Source: CAD feature listing. Evaluate the final solid. Frame: model axes, mm. A direction names the side the tool comes from. Coordinates: 2 decimals unless noted, no trailing zeros. Write each loop counter-clockwise with the first axis right and the second up, starting at its lowest first coordinate (ties: lowest second). Pieces come first, ordered by that corner, then holes. Notation, with made-up numbers: (79, 49) - (131, 49) arc R25 cw to (131, 85) - close; hole circle Ø5 at (-31.5, 29). An arc over 180 degrees is marked (long way). One line per item, written item: value.
from build123d import *

# Parameters (mm, degrees)
SKETCH1_W           = 40
SKETCH1_H           = 10
BOSS_EXTRUDE1_DEPTH = 10
SKETCH2_R           = 2
CUT_EXTRUDE1_DEPTH  = 41
CUT_EXTRUDE2_REACH  = 12
SKETCH3_R           = 0.75


with BuildPart() as part:
    # Sketch1 → Boss-Extrude1 (new body)
    with BuildSketch(Plane(origin=(0, 0, 0), x_dir=(1, 0, 0), z_dir=(0, 1, 0))):
        Rectangle(SKETCH1_W, SKETCH1_H)
    extrude(amount=BOSS_EXTRUDE1_DEPTH)

    # Sketch2 → Cut-Extrude1 (cut, through all)
    with BuildSketch(Plane(origin=(20, 0, 0), x_dir=(0, 0, -1), z_dir=(1, 0, 0))):
        with Locations((0, 4)):
            Circle(SKETCH2_R)
    extrude(amount=-CUT_EXTRUDE1_DEPTH, mode=Mode.SUBTRACT)

    # Sketch3 → Cut-Extrude2 (cut, up to next)
    with BuildSketch(Plane(origin=(0, 10, 0), x_dir=(1, 0, 0), z_dir=(0, 1, 0)), mode=Mode.PRIVATE) as cut_extrude2_sk1:
        with Locations((11, 0)):
            Circle(SKETCH3_R)
    cut_extrude2_tool1 = extrude(cut_extrude2_sk1.sketch, amount=-CUT_EXTRUDE2_REACH, mode=Mode.PRIVATE) & part.part
    add(cut_extrude2_tool1.solids().sort_by_distance((11, 10, 0))[0], mode=Mode.SUBTRACT)
    # Sketch3 → Cut-Extrude2 (cut, up to next)
    with BuildSketch(Plane(origin=(0, 10, 0), x_dir=(1, 0, 0), z_dir=(0, 1, 0)), mode=Mode.PRIVATE) as cut_extrude2_sk2:
        with Locations((6, 0)):
            Circle(SKETCH3_R)
    cut_extrude2_tool2 = extrude(cut_extrude2_sk2.sketch, amount=-CUT_EXTRUDE2_REACH, mode=Mode.PRIVATE) & part.part
    add(cut_extrude2_tool2.solids().sort_by_distance((6, 10, 0))[0], mode=Mode.SUBTRACT)
    # Sketch3 → Cut-Extrude2 (cut, up to next)
    with BuildSketch(Plane(origin=(0, 10, 0), x_dir=(1, 0, 0), z_dir=(0, 1, 0)), mode=Mode.PRIVATE) as cut_extrude2_sk3:
        with Locations((1, 0)):
            Circle(SKETCH3_R)
    cut_extrude2_tool3 = extrude(cut_extrude2_sk3.sketch, amount=-CUT_EXTRUDE2_REACH, mode=Mode.PRIVATE) & part.part
    add(cut_extrude2_tool3.solids().sort_by_distance((1, 10, 0))[0], mode=Mode.SUBTRACT)


solid = part.part
1) Reachability of faces 1 (the flat face through (-20, 6, -1)), 2 (the cylindrical face through (10.25, 7.96, -0.03)) from +Z, -Z, +X, -X, +Y, -Y: full face, straight path, thin tool, end or side. Return the list, or none.
Values found:
face 1: +Z, -Z, -X, +Y, -Y
face 2: +Y
2) Section query A-A on y = 4. Output: boundary loops of the cut face in (x, z).
Values found:
outline: (-20, -5) - (20, -5) - (20, -2) - (-20, -2) - close; (-20, 2) - (20, 2) - (20, 5) - (-20, 5) - close
3) Contact query for flat-ended pins moving along their axis: P1, Ø1.4, axis at x = 6, z = 0, coming from the +Y side; P2, Ø1.7, axis at x = 11, z = 0, coming from the -Y side. Output: stop coordinate, or through.
Values found:
P1: y = 2.13
P2: y = 0
4) Section query B-B on x = -8.5. Output: boundary loops of the cut face in (y, z).
Values found:
outline: (0, -5) - (10, -5) - (10, 5) - (0, 5) - close; hole circle Ø4 at (4, 0)
5) Draft query along Z for faces 3 (the cylindrical face through (0.25, 7.96, -0.03)), 4 (the flat face through (20, 6, -1)), 5 (the cylindrical face through (5.25, 7.96, -0.03)), 6 (the flat face through (0, 5, -5)). Return one class per face: released by +Z, released by -Z, zero draft, split by the parting line, or undercut.
Values found:
face 3: undercut
face 4: zero draft
face 5: undercut
face 6: released by -Z
6) Section query C-C on x = 1. Output: boundary loops of the cut face in (y, z), then the cut area to 3 significant figures.
Values found:
outline: (0, -5) - (10, -5) - (10, -0.75) - (5.85, -0.75) arc R2 cw (long way) to (5.85, 0.75) - (10, 0.75) - (10, 5) - (0, 5) - close
area: 81.4 mm2
7) Material intervals for line 1 (Z direction, x = 1, y = 6.8); line 2 (Y direction, x = 0, z = 1.25); line 3 (Z direction, x = -18, y = 2.25), sorted ascending.
Values found:
line 1: -5 to -0.75, 0.75 to 5
line 2: 0 to 2.44, 5.56 to 10
line 3: -5 to -0.97, 0.97 to 5
